Read the model definition and answer for the solid it produces. Units are mm, in the model's axes. Face numbers are marked on the shaded views. Give positions to 0.01 mm unless a question says otherwise; leave off trailing zeros. Write each loop counter-clockwise with the first axis right and the second up, starting at its lowest first coordinate (ties: lowest second). Pieces come first, ordered by that corner, then holes.
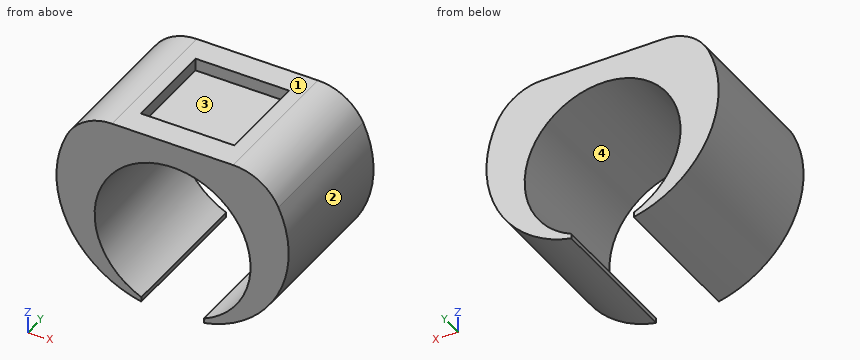
```python
from build123d import *

# Parameters (mm, degrees)
F1_DEPTH = 29.464
F2_R     = 10.16
F3_W     = 19.05
F3_H     = 19.05
F4_DEPTH = 2.54


with BuildPart() as f1:
    # F0 (on Front) → F1 (new body)
    with BuildSketch(Plane.XZ):
        with BuildLine():
            Line((17.4625, 2.54), (-17.4625, 2.54))
            ThreePointArc((-17.4625, 2.54), (-22.643836, -18.887087), (-6.35, -33.735563))
            Line((-6.35, -33.735563), (-6.35, -32.769032))
            ThreePointArc((-6.35, -32.769032), (0, -2.424034), (6.35, -32.769032))
            Line((6.35, -32.769032), (6.35, -33.735565))
            ThreePointArc((6.35, -33.735565), (22.643841, -18.88709), (17.4625, 2.54))
        make_face()
    extrude(amount=F1_DEPTH)

    # F2
    f2_edges = [f1.edges().sort_by_distance(p)[0] for p in [
        (-17.4625, -14.732, 2.54),
        (17.4625, -14.732, 2.54),
    ]]
    fillet(f2_edges, radius=F2_R)

    # F3 (on face) → F4 (cut)
    with BuildSketch(Plane.XY.offset(2.54)):
        with Locations((-0.005137, -14.732)):
            Rectangle(F3_W, F3_H)
    extrude(amount=-F4_DEPTH, mode=Mode.SUBTRACT)


solid = f1.part
```
Item 1: Each of these flat-tipped pins is pushed along its axis until it touches: pin 1 Ø4 at (x, y) = (7.5, -24) entering from -Z; pin 2 Ø3 at (y, z) = (-18.5, 0.5) entering from +X; pin 3 Ø0.8 at (y, z) = (-12, 0.5) entering from -X. Where does it stop, or does it pass through?
Result set:
pin 1: stops at z = -33.74
pin 2: stops at x = 20.03
pin 3: stops at x = -18.93
Item 2: Section C-C (x = 0) is taken. Write down the section's boundary in (y, z).
Result set:
outline: (-29.46, -2.42) - (0, -2.42) - (0, 2.54) - (-5.21, 2.54) - (-5.21, 0) - (-24.26, 0) - (-24.26, 2.54) - (-29.46, 2.54) - close
Item 3: Section A-A (z = -19) is taken. Write down the section's boundary in (x, y).
Result set:
outline: (-22.61, -29.46) - (-15.82, -29.46) - (-15.82, 0) - (-22.61, 0) - close; (15.82, -29.46) - (22.61, -29.46) - (22.61, 0) - (15.82, 0) - close
Item 4: Section D-D (x = -13) is taken. Write down the section's boundary in (y, z), and give its area (3 significant figures).
Result set:
outline: (-29.46, -31.16) - (0, -31.16) - (0, -27.31) - (-29.46, -27.31) - close; (-29.46, -9.22) - (0, -9.22) - (0, 2.52) - (-29.46, 2.52) - close
area: 459 mm2
Item 5: Determine the mould class of the marked faces 1, 2, 3 and 4 for opening direction X: pulls with the +X half, pulls with the -X half, needs draft (parallel to the pull), parting line crosses it, or undercut.
Result set:
face 1: needs draft
face 2: pulls with the +X half
face 3: undercut
face 4: undercut
Item 6: Section B-B (y = -12.5) is taken. Write down the section's boundary in (x, z), and give its area (3 significant figures).
Result set:
outline: (-21.5, -3.26) arc R21.64 ccw to (-6.35, -33.74) - (-6.35, -32.77) arc R15.84 cw (long way) to (6.35, -32.77) - (6.35, -33.74) arc R21.64 ccw to (21.5, -3.26) arc R10.16 ccw to (12.32, 2.54) - (9.52, 2.54) - (9.52, 0) - (-9.53, 0) - (-9.53, 2.54) - (-12.32, 2.54) arc R10.16 ccw to start
area: 623 mm2
Item 7: Find the intervals of material crossed by line 1 along Z through (x, y) = (0, -19.75); line 2 along X through (y, z) = (-26.75, -17.5); line 3 along X through (y, z) = (-25.5, -11.5), in increasing order.
Result set:
line 1: z = -2.42 to 0
line 2: x = -23.02 to -15.82, 15.82 to 23.02
line 3: x = -23.57 to -14.32, 14.32 to 23.57
